Can you work these out from the model? Positions are in its coordinate system, mm. Coordinates: 2 decimals unless noted, no trailing zeros. Loops run counter-clockwise (first coordinate to the right, second up) from the corner with the lowest first, then second, coordinate; pieces in that order, holes last. Notation, with made-up numbers: M -24,-35 L -8,-35 A10 ccw -8,-25 Z; hole C -20.5,9 d11. An arc over 180 degrees is marked long. Answer as a JSON object with one key per item and string values. Group by question number.
Item 1: Suppose I cut it at B-B (x = 6). Write out the boundary of the cut face in (y, z).
Item 2: Suppose I cut it at C-C (z = 7). Write out the boundary of the cut face in (x, y), then the cut area to 3 significant figures.
Item 3: If I drill on line 1 (X direction, y = 0.85, z = 15.25); line 2 (X direction, y = -0.75, z = 6.5); line 3 (Y direction, x = 17, z = 4), over which ranges is the centre line in solid material (lowest first)?
Item 4: Suppose I cut it at A-A (y = -2). Write out the boundary of the cut face in (x, z).
Item 5: Suppose I cut it at D-D (y = 3). Write out the boundary of the cut face in (x, z), then the cut area to 3 significant figures.
Item 6: I'm going to push flat-ended pins straight in: pin 1 Ø2.5 at (x, y) = (-14, -1.5) entering from +Z; pin 2 Ø1.7 at (y, z) = (3, 4.5) entering from +X; pin 3 Ø2.5 at (x, y) = (-17.5, -2) entering from -Z; pin 4 Ø2.5 at (x, z) = (15.25, -15.25) entering from -Y. Where does each tip first touch, or does it pass through?
```python
from build123d import *

# Parameters (mm, degrees)
SZKIC1_R                    = 2
DODANIE_WYCI_GNI_CIE1_DEPTH = 1.8
DODANIE_WYCI_GNI_CIE2_DEPTH = 3.1
ZAOKR_GLENIE1_R             = 1
DODANIE_WYCI_GNI_CIE3_DEPTH = 3.1


with BuildPart() as part:
    # Szkic1 → Dodanie-wyciągnięcie1 (new body)
    with BuildSketch(Plane(origin=(0, 0, 0), x_dir=(1, 0, 0), z_dir=(0, 1, 0))):
        with BuildLine():
            Line((-17, -21.3), (-12.8, -21.3))
            ThreePointArc((-12.8, -21.3), (-10.678679656, -22.178679656), (-9.8, -24.3))
            Line((-9.8, -24.3), (9.8, -24.3))
            ThreePointArc((9.8, -24.3), (10.678679656, -22.178679656), (12.8, -21.3))
            Line((12.8, -21.3), (17, -21.3))
            ThreePointArc((17, -21.3), (20.535533906, -19.835533906), (22, -16.3))
            Line((22, -16.3), (22, 16.3))
            ThreePointArc((22, 16.3), (20.535533906, 19.835533906), (17, 21.3))
            Line((17, 21.3), (12.457318825, 21.3))
            ThreePointArc((12.457318825, 21.3), (11.764572554, 19.361030183), (10, 18.3))
            Line((10, 18.3), (-10, 18.3))
            ThreePointArc((-10, 18.3), (-11.764572554, 19.361030183), (-12.457318825, 21.3))
            Line((-12.457318825, 21.3), (-17, 21.3))
            ThreePointArc((-17, 21.3), (-20.535533906, 19.835533906), (-22, 16.3))
            Line((-22, 16.3), (-22, -16.3))
            ThreePointArc((-22, -16.3), (-20.535533906, -19.835533906), (-17, -21.3))
        make_face()
        with Locations(Location((15.25, 15.25, 0), (0, 0, 270))):
            Circle(SZKIC1_R, mode=Mode.SUBTRACT)
        with Locations(Location((15.25, -15.25, 0), (0, 0, 270))):
            Circle(SZKIC1_R, mode=Mode.SUBTRACT)
        with Locations(Location((-15.25, -15.25, 0), (0, 0, 270))):
            Circle(SZKIC1_R, mode=Mode.SUBTRACT)
        with Locations(Location((-15.25, 15.25, 0), (0, 0, 270))):
            Circle(SZKIC1_R, mode=Mode.SUBTRACT)
    extrude(amount=DODANIE_WYCI_GNI_CIE1_DEPTH)

    # Szkic2 → Dodanie-wyciągnięcie2 (add)
    with BuildSketch(Plane(origin=(0, 1.8, 0), x_dir=(1, 0, 0), z_dir=(0, 1, 0))):
        with BuildLine():
            Line((-10.9, -17.5), (10.9, -17.5))
            ThreePointArc((10.9, -17.5), (12.540202025, -13.540202025), (16.5, -11.9))
            Line((16.5, -11.9), (16.5, 11.9))
            ThreePointArc((16.5, 11.9), (12.540202025, 13.540202025), (10.9, 17.5))
            Line((10.9, 17.5), (-10.9, 17.5))
            ThreePointArc((-10.9, 17.5), (-12.540202025, 13.540202025), (-16.5, 11.9))
            Line((-16.5, 11.9), (-16.5, -11.9))
            ThreePointArc((-16.5, -11.9), (-12.540202025, -13.540202025), (-10.9, -17.5))
        make_face()
    extrude(amount=DODANIE_WYCI_GNI_CIE2_DEPTH)

    # Zaokrąglenie1
    zaokr_glenie1_edges = [part.edges().sort_by_distance(p)[0] for p in [
        (-12.540202025, 4.9, 13.540202025),
        (0, 4.9, 17.5),
        (12.540202025, 4.9, 13.540202025),
        (16.5, 4.9, 0),
        (12.540202025, 4.9, -13.540202025),
        (0, 4.9, -17.5),
        (-12.540202025, 4.9, -13.540202025),
        (-16.5, 4.9, 0),
    ]]
    fillet(zaokr_glenie1_edges, radius=ZAOKR_GLENIE1_R)

    # Szkic3 → Dodanie-wyciągnięcie3 (add)
    with BuildSketch(Plane.XZ):
        Polygon((-12, 17), (12, 17), (12, 12), (20, 12), (20, -12), (12, -12), (12, -17), (-12, -17), (-12, -12), (-20, -12), (-20, 12), (-12, 12), align=None)
    extrude(amount=DODANIE_WYCI_GNI_CIE3_DEPTH)


solid = part.part
```
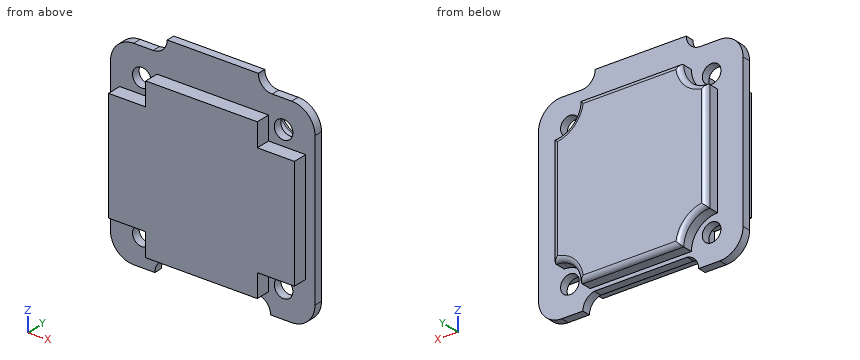
From the geometry:
{
 "1": {"outline": "M -3.1,-17 L 0,-17 L 0,-18.3 L 1.8,-18.3 L 1.8,-17.5 L 3.9,-17.5 A1 ccw 4.9,-16.5 L 4.9,16.5 A1 ccw 3.9,17.5 L 1.8,17.5 L 1.8,24.3 L 0,24.3 L 0,17 L -3.1,17 Z"},
 "2": {"outline": "M -22,0 L -20,0 L -20,-3.1 L 20,-3.1 L 20,0 L 22,0 L 22,1.8 L 16.5,1.8 L 16.5,3.9 A1 ccw 15.5,4.9 L -15.5,4.9 A1 ccw -16.5,3.9 L -16.5,1.8 L -22,1.8 Z", "area": "305 mm2"},
 "3": {"line 1": "-22 to -17.25, -13.25 to 13.25, 17.25 to 22", "line 2": "-20 to 20", "line 3": "-3.1 to 1.8"},
 "4": {"outline": "M -20,-12 L -12,-12 L -12,-17 L 12,-17 L 12,-12 L 20,-12 L 20,12 L 12,12 L 12,17 L -12,17 L -12,12 L -20,12 Z"},
 "5": {"outline": "M -16.5,-11.9 A5.6 cw -10.9,-17.5 L 10.9,-17.5 A5.6 cw 16.5,-11.9 L 16.5,11.9 A5.6 cw 10.9,17.5 L -10.9,17.5 A5.6 cw -16.5,11.9 Z", "area": "1,060 mm2"},
 "6": {"pin 1": "z = 12", "pin 2": "x = 16.5", "pin 3": "z = -12", "pin 4": "through"}
}
